Geometry check sheet. Reference: the model listing, model coordinates, mm. Face numbers are marked on the shaded views. Give positions to 0.01 mm unless a question says otherwise; leave off trailing zeros. Write each loop counter-clockwise with the first axis right and the second up, starting at its lowest first coordinate (ties: lowest second). Pieces come first, ordered by that corner, then holes. Notation, with made-up numbers: M 1.5,83.25 L 17.5,83.25 A25 ccw 17.5,103.25 Z; hole C 81,-27.75 d1. An arc over 180 degrees is marked long. One line per item, written item: value. Start each with the question number.
1. Gauge pin test, flat ends, axial feed: pin 1 (1 mm diameter, centred on x = -4, y = 28, fed in from +Z); pin 2 (8 mm diameter, centred on y = 34, z = 45.5, fed in from +X); pin 3 (1.5 mm diameter, centred on x = -6.5, y = 28, fed in from -Z); pin 4 (3.5 mm diameter, centred on y = 40.07, z = 29.84, fed in from +X). Record the tip position at first contact, or that the pin passes through.
2. Release check for a two-part mould opening along Y. For the marked faces 1, 2 and 3 record: pulls with the +Y half, pulls with the -Y half, needs draft (parallel to the pull), parting line crosses it, or undercut.
3. Cross-section at A-A on y = 25.5. Record the cut outline in (x, z).
4. Scan lines: line 1 (Z direction, x = -5.75, y = 25.5); line 2 (Z direction, x = -5.65, y = 26); line 3 (Y direction, x = -7, z = 79). Record each from-to range of solid material in increasing order.
5. Cross-section at C-C on z = 41.5. Record the cut outline in (x, y) (3 decimals).
6. Cross-section at B-B on x = -4.1. Count the separate pieces of the cut face and the enclosed holes in it, then the cut area to 3 significant figures.
from build123d import *

# Parameters (mm, degrees)
SKETCH1_R           = 2
BOSS_EXTRUDE1_DEPTH = 5
SKETCH2_R           = 2
BOSS_EXTRUDE2_DEPTH = 5


with BuildPart() as part:
    # Sketch1 → Boss-Extrude1 (new body)
    with BuildSketch(Plane(origin=(-2.712826585, 0, 0), x_dir=(0, 0, -1), z_dir=(1, 0, 0))):
        with BuildLine():
            ThreePointArc((-81.47562753, 41.343615563), (-81.034251259, 39.725922602), (-79.907831624, 38.483778355))
            ThreePointArc((-79.907831624, 38.483778355), (-80.372835078, 37.880397724), (-80.772113271, 37.231650221))
            ThreePointArc((-80.772113271, 37.231650221), (-82.332972226, 37.844400456), (-84.002055602, 37.683452608))
            ThreePointArc((-84.002055602, 37.683452608), (-84.100262161, 37.43424746), (-84.192007076, 37.182591734))
            ThreePointArc((-84.192007076, 37.182591734), (-83.049408394, 35.955313535), (-81.474760125, 35.378922733))
            ThreePointArc((-81.474760125, 35.378922733), (-81.606095275, 34.628557837), (-81.65815056, 33.868566623))
            ThreePointArc((-81.65815056, 33.868566623), (-83.324981759, 33.685762686), (-84.728085497, 32.767588723))
            ThreePointArc((-84.728085497, 32.767588723), (-84.69923168, 32.50128966), (-84.663517521, 32.235823593))
            ThreePointArc((-84.663517521, 32.235823593), (-83.081452015, 31.6801148), (-81.419308055, 31.901521629))
            ThreePointArc((-81.419308055, 31.901521629), (-81.1868876, 31.176072024), (-80.879794738, 30.478941927))
            ThreePointArc((-80.879794738, 30.478941927), (-82.270747242, 29.542461997), (-83.086437186, 28.077404509))
            ThreePointArc((-83.086437186, 28.077404509), (-82.937133053, 27.855017437), (-82.782141503, 27.636556105))
            ThreePointArc((-82.782141503, 27.636556105), (-81.123041315, 27.879722907), (-79.754178815, 28.848205731))
            ThreePointArc((-79.754178815, 28.848205731), (-79.211247481, 28.313863177), (-78.615357745, 27.839298301))
            ThreePointArc((-78.615357745, 27.839298301), (-79.411781098, 26.363678645), (-79.45319251, 24.687364646))
            ThreePointArc((-79.45319251, 24.687364646), (-79.217641841, 24.559835763), (-78.978879596, 24.438426025))
            ThreePointArc((-78.978879596, 24.438426025), (-77.622824585, 25.424761837), (-76.860833445, 26.918452913))
            ThreePointArc((-76.860833445, 26.918452913), (-76.131770258, 26.697628851), (-75.383594806, 26.55434629))
            ThreePointArc((-75.383594806, 26.55434629), (-75.403038015, 24.877633587), (-74.660684041, 23.374086413))
            ThreePointArc((-74.660684041, 23.374086413), (-74.392848655, 23.370631049), (-74.125013268, 23.374086413))
            ThreePointArc((-74.125013268, 23.374086413), (-73.382659294, 24.877633587), (-73.402102503, 26.55434629))
            ThreePointArc((-73.402102503, 26.55434629), (-72.653927052, 26.697628851), (-71.924863864, 26.918452913))
            ThreePointArc((-71.924863864, 26.918452913), (-71.162872724, 25.424761837), (-69.806817713, 24.438426025))
            ThreePointArc((-69.806817713, 24.438426025), (-69.568055468, 24.559835763), (-69.332504799, 24.687364646))
            ThreePointArc((-69.332504799, 24.687364646), (-69.373916212, 26.363678645), (-70.170339564, 27.839298301))
            ThreePointArc((-70.170339564, 27.839298301), (-69.574449829, 28.313863177), (-69.031518494, 28.848205731))
            ThreePointArc((-69.031518494, 28.848205731), (-67.662655994, 27.879722907), (-66.003555806, 27.636556105))
            ThreePointArc((-66.003555806, 27.636556105), (-65.848564256, 27.855017437), (-65.699260124, 28.077404509))
            ThreePointArc((-65.699260124, 28.077404509), (-66.514950067, 29.542461997), (-67.905902571, 30.478941927))
            ThreePointArc((-67.905902571, 30.478941927), (-67.598809709, 31.176072024), (-67.366389254, 31.901521629))
            ThreePointArc((-67.366389254, 31.901521629), (-65.704245294, 31.6801148), (-64.122179788, 32.235823593))
            ThreePointArc((-64.122179788, 32.235823593), (-64.086465629, 32.50128966), (-64.057611812, 32.767588723))
            ThreePointArc((-64.057611812, 32.767588723), (-65.46071555, 33.685762686), (-67.12754675, 33.868566623))
            ThreePointArc((-67.12754675, 33.868566623), (-67.179602034, 34.628557837), (-67.310937184, 35.378922733))
            ThreePointArc((-67.310937184, 35.378922733), (-65.736288915, 35.955313535), (-64.593690233, 37.182591734))
            ThreePointArc((-64.593690233, 37.182591734), (-64.685435149, 37.43424746), (-64.783641707, 37.683452608))
            ThreePointArc((-64.783641707, 37.683452608), (-66.452725084, 37.844400456), (-68.013584038, 37.231650221))
            ThreePointArc((-68.013584038, 37.231650221), (-68.412862231, 37.880397724), (-68.877865686, 38.483778355))
            ThreePointArc((-68.877865686, 38.483778355), (-67.75144605, 39.725922602), (-67.31006978, 41.343615563))
            ThreePointArc((-67.31006978, 41.343615563), (-67.508256115, 41.523809654), (-67.711025111, 41.69883099))
            ThreePointArc((-67.711025111, 41.69883099), (-69.263721238, 41.065681511), (-70.361033972, 39.797750798))
            ThreePointArc((-70.361033972, 39.797750798), (-71.016065252, 40.186634356), (-71.708210323, 40.504803491))
            ThreePointArc((-71.708210323, 40.504803491), (-71.288068484, 42.128140906), (-71.64902861, 43.765654666))
            ThreePointArc((-71.64902861, 43.765654666), (-71.908254264, 43.833106827), (-72.169133764, 43.893849073))
            ThreePointArc((-72.169133764, 43.893849073), (-73.249738671, 42.611649181), (-73.632124061, 40.979005638))
            ThreePointArc((-73.632124061, 40.979005638), (-74.392848655, 41.018936713), (-75.153573248, 40.979005638))
            ThreePointArc((-75.153573248, 40.979005638), (-75.535958638, 42.611649181), (-76.616563545, 43.893849073))
            ThreePointArc((-76.616563545, 43.893849073), (-76.877443045, 43.833106827), (-77.1366687, 43.765654666))
            ThreePointArc((-77.1366687, 43.765654666), (-77.497628825, 42.128140906), (-77.077486986, 40.504803491))
            ThreePointArc((-77.077486986, 40.504803491), (-77.769632058, 40.186634356), (-78.424663337, 39.797750798))
            ThreePointArc((-78.424663337, 39.797750798), (-79.521976071, 41.065681511), (-81.074672198, 41.69883099))
            ThreePointArc((-81.074672198, 41.69883099), (-81.277441194, 41.523809654), (-81.47562753, 41.343615563))
        make_face()
        with Locations((-74.392848655, 33.752711127)):
            Circle(SKETCH1_R, mode=Mode.SUBTRACT)
    extrude(amount=-BOSS_EXTRUDE1_DEPTH)

    # Sketch2 → Boss-Extrude2 (add)
    with BuildSketch(Plane(origin=(-2.712826585, 0, 0), x_dir=(0, 0, -1), z_dir=(1, 0, 0))):
        with BuildLine():
            Line((-74.813866248, 36.72302158), (-30.259209457, 43.038285487))
            ThreePointArc((-30.259209457, 43.038285487), (-26.867881411, 40.488992628), (-29.41717427, 37.097664581))
            Line((-29.41717427, 37.097664581), (-73.971831061, 30.782400674))
            ThreePointArc((-73.971831061, 30.782400674), (-71.422538202, 34.173728721), (-74.813866248, 36.72302158))
        make_face()
        with Locations((-29.838191863, 40.067975034)):
            Circle(SKETCH2_R, mode=Mode.SUBTRACT)
    extrude(amount=-BOSS_EXTRUDE2_DEPTH)


solid = part.part
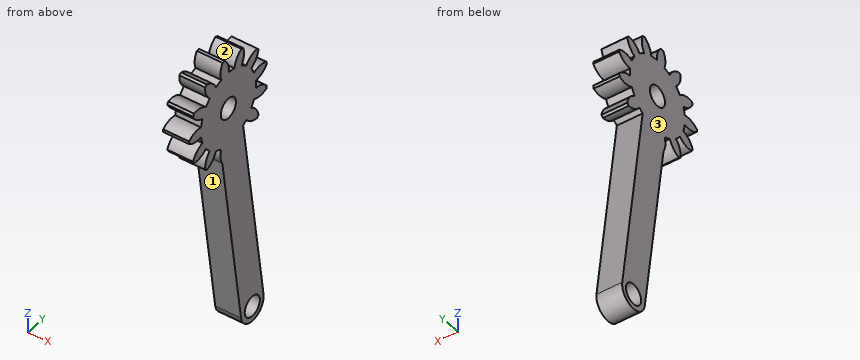
Report:
1. pin 1: stops at z = 83.09
1. pin 2: stops at x = -2.71
1. pin 3: stops at z = 65.7
1. pin 4: passes through
2. face 1: pulls with the -Y half
2. face 2: undercut
2. face 3: needs draft
3. outline: M -7.71,69.25 L -2.71,69.25 L -2.71,71.23 L -7.71,71.23 Z; M -7.71,73.3 L -2.71,73.3 L -2.71,75.49 L -7.71,75.49 Z; M -7.71,77.56 L -2.71,77.56 L -2.71,79.53 L -7.71,79.53 Z
4. line 1: z = 69.25 to 71.23, 73.3 to 75.49, 77.56 to 79.53
4. line 2: z = 69.3 to 71.56, 73.31 to 75.48, 77.22 to 79.49
4. line 3: y = 24.45 to 27.32, 28.13 to 40.61
5. outline: M -7.713,35.385 L -2.713,35.385 L -2.713,41.445 L -7.713,41.445 Z
6. separate pieces: 1
6. enclosed holes: 2
6. area: 445 mm^2
